Design review of the part shown in the three views and the two pictorial views. Dimensions are in mm from the part's minimum x, y and z. Coordinates: 2 decimals unless noted, no trailing zeros. Write each loop counter-clockwise with the first axis right and the second up, starting at its lowest first coordinate (ties: lowest second). Pieces come first, ordered by that corner, then holes. Notation, with made-up numbers: (43.25, 53) -> (69.25, 53) arc R21 cw to (69.25, 66) -> close; hole circle Ø8 at (-10, 81.5). An arc over 180 degrees is marked (long way). Answer in a Markdown table with one row per item. Add a question column.
Item 1: Draft analysis for pull direction Y (two halves, no side actions). For the marked faces 1, 2 and 3, state which applies: released by +Y, released by -Y, zero draft, split by the parting line, or undercut.
Item 2: To check wall thickness, follow line 1 (Y direction, x = 4.5, z = 1.6); line 2 (X direction, y = 3, z = 2.4); line 3 (X direction, y = 2.5, z = 1.1). State the ranges of each line that lie inside material, in increasing order.
Item 3: Clearance check with flat-ended pins moving along their axes: P1, Ø5, axis at x = 4.5, y = 4.5, coming from the +Z side; P2, Ø1.5, axis at x = 3.5, z = 2, coming from the -Y side; P3, Ø1, axis at x = 2.5, z = 2.5, coming from the -Y side; P4, Ø1.5, axis at x = 4.5, y = 7.5, coming from the -Z side. State where each tip first meets the part, or that it passes through.
Item 4: Take a section at C-C, the plane z = 1.75. Write out the cut boundary in (x, y), and give its area (3 significant figures).
Item 5: Take a section at A-A, the plane x = 4.5. Write out the cut boundary in (y, z), and give its area (3 significant figures).
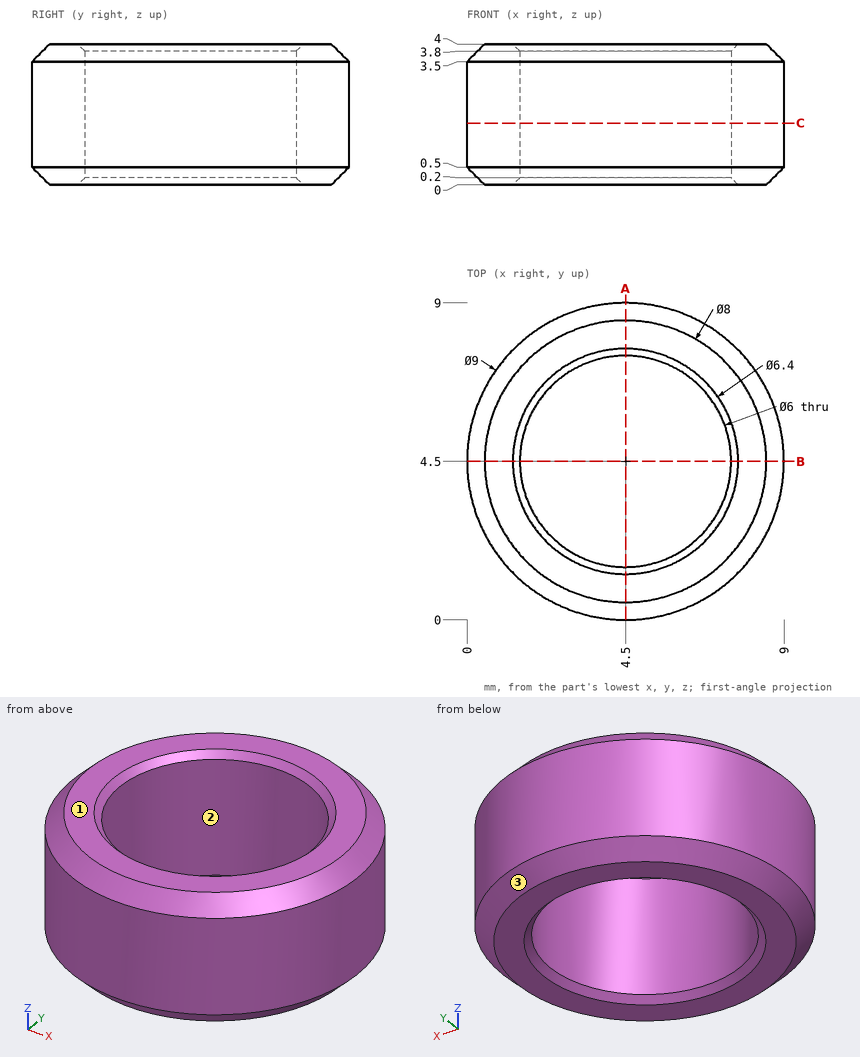
Answers:
| question | item | result |
|---|---|---|
| 1 | face 1 | zero draft |
| 1 | face 2 | undercut |
| 1 | face 3 | split by the parting line |
| 2 | line 1 | y = 0 to 1.5, 7.5 to 9 |
| 2 | line 2 | x = 0.26 to 1.9, 7.1 to 8.74 |
| 2 | line 3 | x = 0.47 to 2.26, 6.74 to 8.53 |
| 3 | P1 | passes through |
| 3 | P2 | stops at y = 0.01 |
| 3 | P3 | stops at y = 0.26 |
| 3 | P4 | stops at z = 0 |
| 4 | outline | circle Ø9 at (4.5, 4.5); hole circle Ø6 at (4.5, 4.5) |
| 4 | area | 35.3 mm^2 |
| 5 | outline | (0, 0.5) -> (0.5, 0) -> (1.3, 0) -> (1.5, 0.2) -> (1.5, 3.8) -> (1.3, 4) -> (0.5, 4) -> (0, 3.5) -> close; (7.5, 0.2) -> (7.7, 0) -> (8.5, 0) -> (9, 0.5) -> (9, 3.5) -> (8.5, 4) -> (7.7, 4) -> (7.5, 3.8) -> close |
| 5 | area | 11.4 mm^2 |
